from build123d import *

# Parameters (mm, degrees)
SKETCH2_R          = 2.9
CUT_EXTRUDE1_DEPTH = 13
FILLET1_R          = 1


with BuildPart() as part:
    # Sketch1 → Revolve1 (revolve)
    with BuildSketch(Plane.XY, mode=Mode.PRIVATE) as revolve1_sk:
        Polygon((0, 0), (20, 0), (0, 25), align=None)
    revolve(revolve1_sk.sketch.rotate(Axis((0, 25, 0), (0, -1, 0)), 270), axis=Axis((0, 25, 0), (0, -1, 0)))

    # Sketch2 → Cut-Extrude1 (cut)
    with BuildSketch(Plane.XZ):
        with Locations(Location((0, 0, 0), (0, 0, 270))):
            Circle(SKETCH2_R)
    extrude(amount=-CUT_EXTRUDE1_DEPTH, mode=Mode.SUBTRACT)

    # Fillet1
    fillet1_edges = [part.edges().sort_by_distance(p)[0] for p in [
        (0, 0, 20),
    ]]
    fillet(fillet1_edges, radius=FILLET1_R)


solid = part.part
Model file for the job. Use its own axes, mm. Round coordinates to 2 decimals unless told otherwise and drop trailing zeros. Order: outer loops, then holes, each group sorted by start corner. A loop starts at its lowest first (then second) coordinate and runs counter-clockwise, first axis right, second up.
(1) Band-saw the part on A-A (y = 5.25). List the corners of the cut face in (x, z).
(2) Drill centre lines: line 1 (X direction, y = 9.75, z = 0); line 2 (X direction, y = 5.5, z = 0); line 3 (Z direction, x = 2.5, y = 1.5). Where is each one in solid material? Low to high.
(3) Band-saw the part on B-B (y = 16.5). List the corners of the cut face in (x, z), then the cut area to 3 significant figures.
(4) Pull direction X, two halves, no side cores. Call faces 1 (the face through (-4, 0, 0)), 2 (the face through (0, 13, 0)), 3 (the face through (1.52, 18.67, -4.83)): released by +X, released by -X, zero draft, split by the parting line, or undercut.
(5) Pin check, flat tips, straight feed: pin 1 (4 mm diameter, centred on y = 4, z = -4.5, fed in from -X); pin 2 (1 mm diameter, centred on y = 4, z = 10, fed in from +X); pin 3 (2 mm diameter, centred on y = 3, z = 11, fed in from -X). Stop position of each tip, or through.
(6) Band-saw the part on C-C (y = 2.75). List the corners of the cut face in (x, z).
Verdict:
1. outline: circle Ø31.6 at (0, 0); hole circle Ø5.8 at (0, 0)
2. line 1: x = -12.2 to -2.9, 2.9 to 12.2
2. line 2: x = -15.6 to -2.9, 2.9 to 15.6
2. line 3: z = -18.62 to -1.47, 1.47 to 18.62
3. outline: circle Ø13.6 at (0, 0)
3. area: 145 mm2
4. face 1: zero draft
4. face 2: undercut
4. face 3: split by the parting line
5. pin 1: stops at x = -17.91
5. pin 2: stops at x = 14.11
5. pin 3: stops at x = -14.98
6. outline: circle Ø35.6 at (0, 0); hole circle Ø5.8 at (0, 0)
